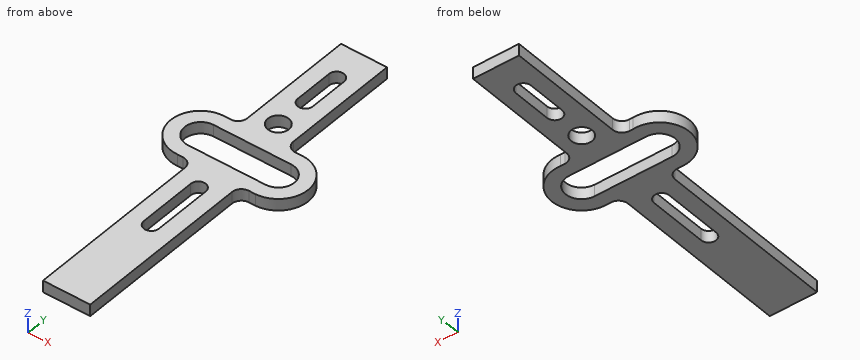
```python
from build123d import *

# Parameters (mm, degrees)
BOSS_EXTRUDE1_DEPTH = 2.997
SKETCH2_R           = 2.6925
CUT_EXTRUDE1_DEPTH  = 99.123678721
CUT_EXTRUDE2_DEPTH  = 99.123678721
CUT_EXTRUDE3_DEPTH  = 99.123678721
CUT_EXTRUDE4_DEPTH  = 99.123678721


with BuildPart() as part:
    # Sketch1 → Boss-Extrude1 (new body)
    with BuildSketch(Plane.XY):
        with BuildLine():
            Line((0, 0), (12.08, 0))
            Line((12.08, 0), (12.08, 45.311))
            ThreePointArc((12.08, 45.311), (12.777378754, 46.994621246), (14.461, 47.692))
            Line((14.461, 47.692), (16.139481493, 47.692))
            ThreePointArc((16.139481493, 47.692), (23.535730768, 55.74130609), (15.275362275, 62.901064761))
            Line((15.275362275, 62.901064761), (14.141, 62.901064761))
            ThreePointArc((14.141, 62.901064761), (12.457378754, 63.598443515), (11.76, 65.282064761))
            Line((11.76, 65.282064761), (11.76, 95.209064761))
            Line((11.76, 95.209064761), (0, 95.209064761))
            Line((0, 95.209064761), (0, 65.282064761))
            ThreePointArc((0, 65.282064761), (-0.697378754, 63.598443515), (-2.381, 62.901064761))
            Line((-2.381, 62.901064761), (-3.358362275, 62.901064761))
            ThreePointArc((-3.358362275, 62.901064761), (-11.627796455, 55.52999861), (-3.799518507, 47.692))
            Line((-3.799518507, 47.692), (-2.381, 47.692))
            ThreePointArc((-2.381, 47.692), (-0.697378754, 46.994621246), (0, 45.311))
            Line((0, 45.311), (0, 0))
        make_face()
    extrude(amount=BOSS_EXTRUDE1_DEPTH)

    # Sketch2 → Cut-Extrude1 (cut, through all)
    with BuildSketch(Plane.XY.offset(2.997)):
        with Locations((5.959, 67.726064761)):
            Circle(SKETCH2_R)
    extrude(amount=-CUT_EXTRUDE1_DEPTH, mode=Mode.SUBTRACT)

    # Sketch3 → Cut-Extrude2 (cut, through all)
    with BuildSketch(Plane.XY.offset(2.997)):
        with BuildLine():
            Line((-3.970876758, 59.441), (15.890123242, 59.441))
            ThreePointArc((15.890123242, 59.441), (19.979623242, 55.3515), (15.890123242, 51.262))
            Line((15.890123242, 51.262), (-3.970876758, 51.262))
            ThreePointArc((-3.970876758, 51.262), (-8.060376758, 55.3515), (-3.970876758, 59.441))
        make_face()
    extrude(amount=-CUT_EXTRUDE2_DEPTH, mode=Mode.SUBTRACT)

    # Sketch4 → Cut-Extrude3 (cut, through all)
    with BuildSketch(Plane.XY.offset(2.997)):
        with BuildLine():
            Line((7.889, 86.344064761), (7.889, 76.362064761))
            ThreePointArc((7.889, 76.362064761), (5.9585, 74.431564761), (4.028, 76.362064761))
            Line((4.028, 76.362064761), (4.028, 86.344064761))
            ThreePointArc((4.028, 86.344064761), (5.9585, 88.274564761), (7.889, 86.344064761))
        make_face()
    extrude(amount=-CUT_EXTRUDE3_DEPTH, mode=Mode.SUBTRACT)

    # Sketch5 → Cut-Extrude4 (cut, through all)
    with BuildSketch(Plane.XY.offset(2.997)):
        with BuildLine():
            Line((7.889, 42.164), (7.889, 27.178))
            ThreePointArc((7.889, 27.178), (5.9585, 25.2475), (4.028, 27.178))
            Line((4.028, 27.178), (4.028, 42.164))
            ThreePointArc((4.028, 42.164), (5.9585, 44.0945), (7.889, 42.164))
        make_face()
    extrude(amount=-CUT_EXTRUDE4_DEPTH, mode=Mode.SUBTRACT)


solid = part.part
```
Geometry: final body of the model. Coordinates: model frame, mm. Coordinates: 2 decimals unless noted, no trailing zeros. Order: outer loops, then holes, each group sorted by start corner. A loop starts at its lowest first (then second) coordinate and runs counter-clockwise, first axis right, second up. Notation, with made-up numbers: (-35.5, 73) -> (-1.5, 73) arc R7 cw to (-1.5, 79) -> close; hole circle Ø11 at (82.25, 40.5). An arc over 180 degrees is marked (long way). Answer in a Markdown table with one row per item.
Item 1: Section B-B on x = 6. Output: boundary loops of the cut face in (y, z), plus the area to 3 significant figures.
Return value:
| item | result |
|---|---|
| outline | (0, 0) -> (25.25, 0) -> (25.25, 3) -> (0, 3) -> close; (44.09, 0) -> (51.26, 0) -> (51.26, 3) -> (44.09, 3) -> close; (59.44, 0) -> (65.03, 0) -> (65.03, 3) -> (59.44, 3) -> close; (70.42, 0) -> (74.43, 0) -> (74.43, 3) -> (70.42, 3) -> close; (88.27, 0) -> (95.21, 0) -> (95.21, 3) -> (88.27, 3) -> close |
| area | 147 mm² |
Item 2: Section C-C on z = 1.75. State how many separate pieces and enclosed holes the cut face has, plus the area to 3 significant figures.
Return value:
| item | result |
|---|---|
| separate pieces | 1 |
| enclosed holes | 4 |
| area | 1,090 mm² |
Item 3: Contact query for flat-ended pins moving along their axis: P1, Ø1.5, axis at y = 36, z = 2, coming from the -X side; P2, Ø1.2, axis at x = 15, z = 1.5, coming from the +Y side; P3, Ø0.7, axis at x = -3, z = 1, coming from the -Y side. Output: stop coordinate, or through.
Return value:
| item | result |
|---|---|
| P1 | stops at x = 0 |
| P2 | stops at y = 62.92 |
| P3 | stops at y = 47.69 |
Item 4: Section A-A on y = 29. Output: boundary loops of the cut face in (x, z), plus the area to 3 significant figures.
Return value:
| item | result |
|---|---|
| outline | (0, 0) -> (4.03, 0) -> (4.03, 3) -> (0, 3) -> close; (7.89, 0) -> (12.08, 0) -> (12.08, 3) -> (7.89, 3) -> close |
| area | 24.6 mm² |
Item 5: Ray query, L1, parallel to Y at x = 6, z = 0.3; L2, parallel to Y at x = 3, z = 1.8; L3, parallel to X at y = 34.5, z = 1.7. Return the intervals inside material, ascending.
Return value:
| item | result |
|---|---|
| L1 | y = 0 to 25.25, 44.09 to 51.26, 59.44 to 65.03, 70.42 to 74.43, 88.27 to 95.21 |
| L2 | y = 0 to 51.26, 59.44 to 95.21 |
| L3 | x = 0 to 4.03, 7.89 to 12.08 |
Item 6: Section D-D on x = 17. Output: boundary loops of the cut face in (y, z), plus the area to 3 significant figures.
Return value:
| item | result |
|---|---|
| outline | (47.76, 0) -> (51.42, 0) -> (51.42, 3) -> (47.76, 3) -> close; (59.29, 0) -> (62.85, 0) -> (62.85, 3) -> (59.29, 3) -> close |
| area | 21.6 mm² |
